```python
from build123d import *

# Parameters (mm, degrees)
BOSS_EXTRUDE1_DEPTH = 5
BOSS_EXTRUDE2_DEPTH = 15
SKETCH3_W           = 50
SKETCH3_H           = 210
BOSS_EXTRUDE3_DEPTH = 50
SKETCH4_W           = 40
SKETCH4_H           = 45
CUT_EXTRUDE2_DEPTH  = 210


with BuildPart() as part:
    # Sketch1 → Boss-Extrude1 (new body)
    with BuildSketch(Plane(origin=(0, 0, 0), x_dir=(1, 0, 0), z_dir=(0, 1, 0))):
        Polygon((-37.5, -105), (37.5, 105), (37.5, -105), align=None)
    extrude(amount=BOSS_EXTRUDE1_DEPTH)

    # Sketch2 → Boss-Extrude2 (add)
    with BuildSketch(Plane(origin=(0, 5, 0), x_dir=(1, 0, 0), z_dir=(0, 1, 0))):
        Polygon((-37.5, -105), (37.5, -105), (37.5, -100), (-35.714285714, -100), align=None)
    extrude(amount=BOSS_EXTRUDE2_DEPTH)

    # Sketch3 → Boss-Extrude3 (add)
    with BuildSketch(Plane.XZ):
        with Locations((62.5, 0)):
            Rectangle(SKETCH3_W, SKETCH3_H)
    extrude(amount=-BOSS_EXTRUDE3_DEPTH)

    # Sketch4 → Cut-Extrude2 (cut)
    with BuildSketch(Plane(origin=(0, 0, -105), x_dir=(-1, 0, 0), z_dir=(0, 0, -1))):
        with Locations((-62.5, 27.5)):
            Rectangle(SKETCH4_W, SKETCH4_H)
    extrude(amount=-CUT_EXTRUDE2_DEPTH, mode=Mode.SUBTRACT)


solid = part.part
```
Part model, mm, in its own coordinate system. A direction names the side the tool comes from. Give positions to 0.01 mm unless a question says otherwise; leave off trailing zeros. Write each loop counter-clockwise with the first axis right and the second up, starting at its lowest first coordinate (ties: lowest second). Pieces come first, ordered by that corner, then holes. Notation, with made-up numbers: M -38.5,-19.5 L 0.5,-19.5 A16 ccw 0.5,-10.5 Z; hole C 6,-39.5 d2. An arc over 180 degrees is marked long. Use CSV: the item, a comma, the result in double quotes.
Item 1: Slice it at D-D on y = 47.5. Write the cut outline in (x, z), plus the area to 3 significant figures.
Taken from the geometry:
outline,"M 37.5,-105 L 42.5,-105 L 42.5,105 L 37.5,105 Z; M 82.5,-105 L 87.5,-105 L 87.5,105 L 82.5,105 Z"
area,"2,100 mm²"
Item 2: Slice it at A-A on y = 17. Write the cut outline in (x, z), plus the area to 3 significant figures.
Taken from the geometry:
outline,"M -37.5,105 L -35.71,100 L 37.5,100 L 37.5,-105 L 42.5,-105 L 42.5,105 Z; M 82.5,-105 L 87.5,-105 L 87.5,105 L 82.5,105 Z"
area,"2,470 mm²"
Item 3: Which spindle directions (+Z, -Z, +X, -X, +Y, -Y) get a long thin tool onto all of the face, cutting with end or side? Do faces 5 (the face through (-1, 20, 102)), 6 (the face through (63, 5, -1)), 7 (the face through (18, 5, 42)). Say none if no direction does.
Taken from the geometry:
face 5,"+Z, -Z, -X, +Y"
face 6,"+Z, -Z, +Y"
face 7,"-Z, -X, +Y"
Item 4: Pull direction X, two halves, no side cores. Call faces 1 (the face through (38, 0, 25)), 2 (the face through (42.5, 27, -1)), 3 (the face through (87.5, 25, -1)), 4 (the face through (82.5, 27, -1)): +X half, -X half, draft (parallel to the pull), parting line (faces both ways), or undercut.
Taken from the geometry:
face 1,"draft"
face 2,"undercut"
face 3,"+X half"
face 4,"undercut"
Item 5: Slice it at B-B on z = -42. Write the cut outline in (x, y), plus the area to 4 significant figures.
Taken from the geometry:
outline,"M 15,0 L 87.5,0 L 87.5,50 L 82.5,50 L 82.5,5 L 42.5,5 L 42.5,50 L 37.5,50 L 37.5,5 L 15,5 Z"
area,"812.5 mm²"
Item 6: Pin check, flat tips, straight feed: P1, Ø5.5, axis at x = -2, z = 102, coming from the +Y side; P2, Ø20, axis at x = 56.5, z = -29.5, coming from the +Y side; P3, Ø22.5, axis at y = 24, z = -3, coming from the -X side. Stop position of each tip, or through.
Taken from the geometry:
P1,"stops at y = 20"
P2,"stops at y = 5"
P3,"stops at x = 37.5"
Item 7: Slice it at C-C on x = -13. Write the cut outline in (y, z), plus the area to 3 significant figures.
Taken from the geometry:
outline,"M 0,36.4 L 5,36.4 L 5,100 L 20,100 L 20,105 L 0,105 Z"
area,"418 mm²"
Item 8: Drill centre lines: probe 1 along X at (y, z) = (47, 38); probe 2 along Y at (x, z) = (11.5, 76); probe 3 along X at (y, z) = (4.5, -41.5). Where is each one in solid material? Low to high.
Taken from the geometry:
probe 1,"x = 37.5 to 42.5, 82.5 to 87.5"
probe 2,"y = 0 to 5"
probe 3,"x = 14.82 to 87.5"
